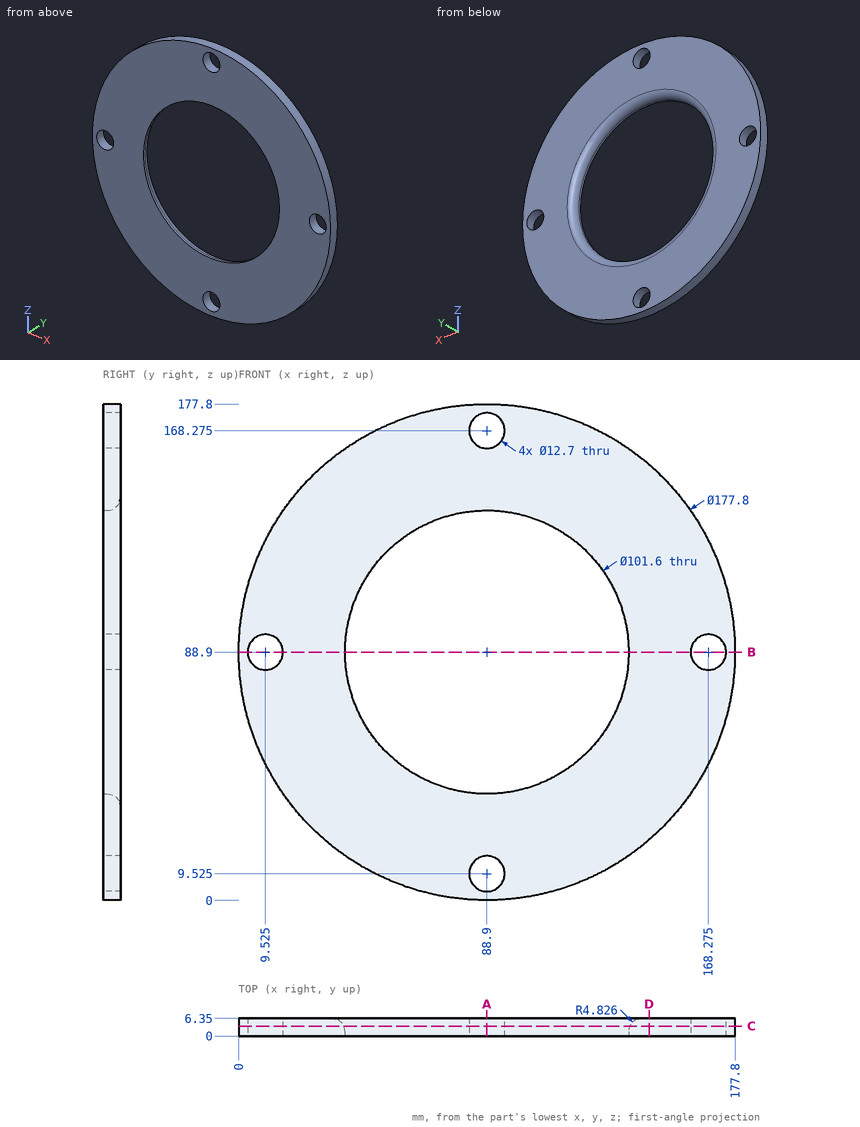
The figure shows three views and two pictorial views of one solid part (mm, origin at its lowest corner). Answer the questions. Round coordinates to 2 decimals unless told otherwise and drop trailing zeros. Write each loop counter-clockwise with the first axis right and the second up, starting at its lowest first coordinate (ties: lowest second). Pieces come first, ordered by that corner, then holes. Notation, with made-up numbers: M 4.5,-13.75 L 29.5,-13.75 A19 cw 29.5,-5.75 Z; hole C -18,5.5 d7. An arc over 180 degrees is marked long. Use a Markdown table: item, result.
1) The part is cut by section C-C (y = 3.5). Write down the section's boundary in (x, z) (3 decimals).
Answers follow:
| item | result |
|---|---|
| outline | C 88.9,88.9 d177.8; hole C 9.525,88.9 d12.7; hole C 88.9,88.9 d102.446; hole C 88.9,9.525 d12.7; hole C 88.9,168.275 d12.7; hole C 168.275,88.9 d12.7 |
2) Flat-ended cylindrical pins translate along their axes: pin 1 (12 mm diameter, centred on x = 138, z = 103, fed in from +Y); pin 2 (1.5 mm diameter, centred on y = 2.5, z = 59.5, fed in from +X). Find the tip coordinate at first contact, or state that the pin passes through.
Answers follow:
| item | result |
|---|---|
| pin 1 | stops at y = 6.35 |
| pin 2 | stops at x = 173.06 |
3) The part is cut by section A-A (x = 88.9). Write down the section's boundary in (y, z) (3 decimals), plus the area to 3 significant figures.
Answers follow:
| item | result |
|---|---|
| outline | M 0,0 L 6.35,0 L 6.35,3.175 L 0,3.175 Z; M 0,15.875 L 6.35,15.875 L 6.35,33.274 A4.826 ccw 1.524,38.1 L 0,38.1 Z; M 0,139.7 L 1.524,139.7 A4.826 ccw 6.35,144.526 L 6.35,161.925 L 0,161.925 Z; M 0,174.625 L 6.35,174.625 L 6.35,177.8 L 0,177.8 Z |
| area | 313 mm2 |
4) The part is cut by section D-D (x = 147). Write down the section's boundary in (y, z).
Answers follow:
| item | result |
|---|---|
| outline | M 0,21.61 L 6.35,21.61 L 6.35,156.19 L 0,156.19 Z |
5) The part is cut by section B-B (z = 88.9). Write down the section's boundary in (x, y) (3 decimals), plus the area to 3 significant figures.
Answers follow:
| item | result |
|---|---|
| outline | M 0,0 L 3.175,0 L 3.175,6.35 L 0,6.35 Z; M 15.875,0 L 38.1,0 L 38.1,1.524 A4.826 ccw 33.274,6.35 L 15.875,6.35 Z; M 139.7,0 L 161.925,0 L 161.925,6.35 L 144.526,6.35 A4.826 ccw 139.7,1.524 Z; M 174.625,0 L 177.8,0 L 177.8,6.35 L 174.625,6.35 Z |
| area | 313 mm2 |
6) Straight lines are drawn through the part: line 1 along Z through (x, y) = (88.9, 1.5) (3 decimals); line 2 along Z through (x, y) = (92, 4.5); line 3 along X through (y, z) = (1.25, 103.5). For each, find the intervals that lie inside material, in ascending order. Write a range as [from, to].
Answers follow:
| item | result |
|---|---|
| line 1 | z = [0, 3.175], [15.875, 38.1], [139.7, 161.925], [174.625, 177.8] |
| line 2 | z = [0.05, 3.98], [15.07, 37.17], [140.63, 162.73], [173.82, 177.75] |
| line 3 | x = [1.21, 40.24], [137.56, 176.59] |
